```python
from build123d import *

# Parameters (mm, degrees)
F2_R = 9.5
F4_R = 9.6520512263


# Not quite as in the source:
# - a fillet or chamfer that OpenCascade refuses, or shapes differently, is made with other operations: its cross-section is extruded or revolved along the edge and cut away or added


with BuildPart() as f1:
    # F0 (on Front) → F1 (revolve)
    with BuildSketch(Plane.XZ):
        Polygon((0, 4), (0, 0), (50, 0), (50, 9.5), (8, 9.5), (8, 4), align=None)
    revolve(axis=Axis((25, 0, 0), (-1, 0, 0)))

    # F2
    f2_edges = [f1.edges().sort_by_distance(p)[0] for p in [
        (50, 0, -9.5),
    ]]
    fillet(f2_edges, radius=F2_R)

    # F3: fillet of radius 8.4497474683 on 1 edges, made by hand

    # F3_s1 → F3_t2 (revolve, cut)
    with BuildSketch(Plane.XZ):
        with BuildLine():
            ThreePointArc((15.9181577498, 9.5), (11.0977007655, 7.990095955), (8, 4))
            Line((8, 4), (8, 9.5))
            Line((8, 9.5), (15.9181577498, 9.5))
        make_face()
    revolve(axis=Axis((8, 0, 0), (-1, 0, 0)), mode=Mode.SUBTRACT)

    # F4
    f4_edges = [f1.edges().sort_by_distance(p)[0] for p in [
        (8, 0, -4),
    ]]
    fillet(f4_edges, radius=F4_R)


solid = f1.part
```
Work out the finished part from the listing and answer in its coordinate system (mm). A direction names the side the tool comes from. Coordinates: 2 decimals unless noted, no trailing zeros. Loops run counter-clockwise (first coordinate to the right, second up) from the corner with the lowest first, then second, coordinate; pieces in that order, holes last. Notation, with made-up numbers: (24.25, 89) - (30.25, 89) arc R19 ccw to (30.25, 95) - close; hole circle Ø10 at (41, 9.5). An arc over 180 degrees is marked (long way). Use a Markdown table: item, result.
Item 1: For faces 1 (the cylindrical face through (1.441, -1.532, 3.695)), 2 (the cylindrical face through (28.04, -8.43, 4.38)), determine the directions among +Z, -Z, +X, -X, +Y, -Y from which every point of the face is accessible in a straight line to the end or side of a thin tool.
Evaluation:
| item | result |
|---|---|
| face 1 | -X |
| face 2 | +X, -X |
Item 2: Find section A-A, the plane x = 25. Determine the outline of the cut face in (y, z), and give its area (3 significant figures).
Evaluation:
| item | result |
|---|---|
| outline | circle Ø19 at (0, 0) |
| area | 284 mm2 |
Item 3: Consider probe 1 along Y at (x, z) = (34, 0); probe 2 along Y at (x, z) = (30.5, -5.75); probe 3 along X at (y, z) = (5, -6.5). Determine where each line is inside the solid, lowest interval first. Write a range as from..to.
Evaluation:
| item | result |
|---|---|
| probe 1 | y = -9.5..9.5 |
| probe 2 | y = -7.56..7.56 |
| probe 3 | x = 11.42..45.3 |
Item 4: Given pin 1 Ø1.5 at (y, z) = (-1.5, -2) entering from -X; pin 2 Ø8 at (y, z) = (2, -5) entering from +X; pin 3 Ø5 at (x, z) = (43.5, -6) entering from +Y; pin 4 Ø1 at (x, z) = (39.5, -4.5) entering from +Y, each flat-ended and moving along its own axis, determine where each tip first touches the part or whether it passes through.
Evaluation:
| item | result |
|---|---|
| pin 1 | stops at x = 0 |
| pin 2 | stops at x = 49.9 |
| pin 3 | stops at y = 8.52 |
| pin 4 | stops at y = 8.62 |
Item 5: Find section B-B, the plane x = 43. Determine the outline of the cut face in (y, z), and give its area (3 significant figures).
Evaluation:
| item | result |
|---|---|
| outline | circle Ø18.33 at (0, 0) |
| area | 264 mm2 |
